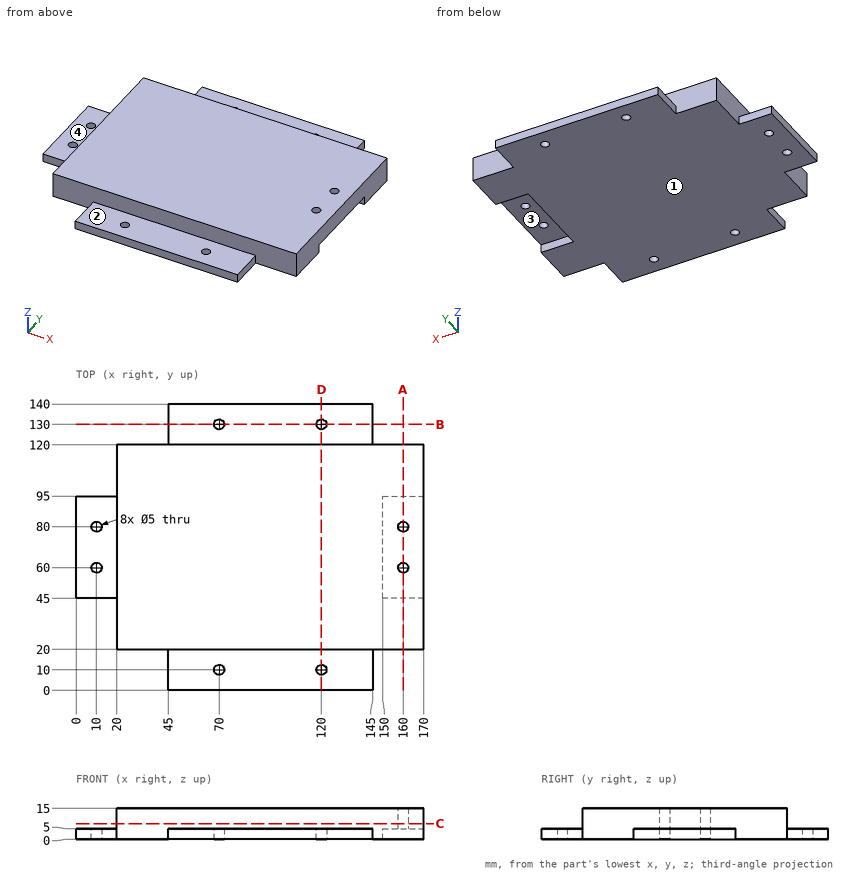
Study the drawing (mm; zero at the part's minimum x, y, z) and answer. A direction names the side the tool comes from. Coordinates: 2 decimals unless noted, no trailing zeros. Write each loop counter-clockwise with the first axis right and the second up, starting at its lowest first coordinate (ties: lowest second). Pieces come first, ordered by that corner, then holes. Notation, with made-up numbers: (9, 54.5) - (67, 54.5) arc R13 ccw to (67, 59.5) - close; hole circle Ø5 at (-5, -36). An arc over 180 degrees is marked (long way). One line per question, with ' | ' between items.
1) Find section B-B, the plane y = 130. Determine the outline of the cut face in (x, z).
Checks:
outline: (45, 0) - (67.5, 0) - (67.5, 5) - (45, 5) - close; (72.5, 0) - (117.5, 0) - (117.5, 5) - (72.5, 5) - close; (122.5, 0) - (145, 0) - (145, 5) - (122.5, 5) - close
2) Find section C-C, the plane z = 7.5. Determine the outline of the cut face in (x, y), and give its area (3 significant figures).
Checks:
outline: (20, 20) - (170, 20) - (170, 120) - (20, 120) - close; hole circle Ø5 at (160, 60); hole circle Ø5 at (160, 80) | area: 15,000 mm2
3) For the marked faces 1 and 2, determine the directions among +Z, -Z, +X, -X, +Y, -Y from which every point of the face is accessible in a straight line to the end or side of a thin tool.
Checks:
face 1: -Z, +X, -X, +Y, -Y | face 2: +Z, +X, -X, -Y
4) Flat-ended cylindrical pins translate along their axes: P1, Ø8, axis at x = 21, z = 2, coming from the +Y side; P2, Ø8, axis at x = 120, y = 130, coming from the +Z side; P3, Ø5.5, axis at x = 8, z = 3.5, coming from the -Y side; P4, Ø4, axis at y = 123.5, z = 12.5, coming from the +X side. Find the tip coordinate at first contact, or state that the pin passes through.
Checks:
P1: y = 120 | P2: z = 5 | P3: y = 45 | P4: through
5) Find section D-D, the plane x = 120. Determine the outline of the cut face in (y, z).
Checks:
outline: (0, 0) - (7.5, 0) - (7.5, 5) - (0, 5) - close; (12.5, 0) - (127.5, 0) - (127.5, 5) - (120, 5) - (120, 15) - (20, 15) - (20, 5) - (12.5, 5) - close; (132.5, 0) - (140, 0) - (140, 5) - (132.5, 5) - close
6) The mould has two halves that part along Y. Classify the marked faces 3 and 4: +Y half, -Y half, draft (parallel to the pull), parting line (faces both ways), or undercut.
Checks:
face 3: undercut | face 4: draft
7) Find section A-A, the plane x = 160. Determine the outline of the cut face in (y, z), and give its area (3 significant figures).
Checks:
outline: (20, 0) - (45, 0) - (45, 5) - (57.5, 5) - (57.5, 15) - (20, 15) - close; (62.5, 5) - (77.5, 5) - (77.5, 15) - (62.5, 15) - close; (82.5, 5) - (95, 5) - (95, 0) - (120, 0) - (120, 15) - (82.5, 15) - close | area: 1,150 mm2
8) Consider probe 1 along Y at (x, z) = (10, 3.85); probe 2 along Y at (x, z) = (120, 1.25); probe 3 along X at (y, z) = (130, 2.4). Determine where each line is inside the solid, lowest interval first. Write a range as [from, to].
Checks:
probe 1: [45, 57.5], [62.5, 77.5], [82.5, 95] | probe 2: [0, 7.5], [12.5, 127.5], [132.5, 140] | probe 3: [45, 67.5], [72.5, 117.5], [122.5, 145]
